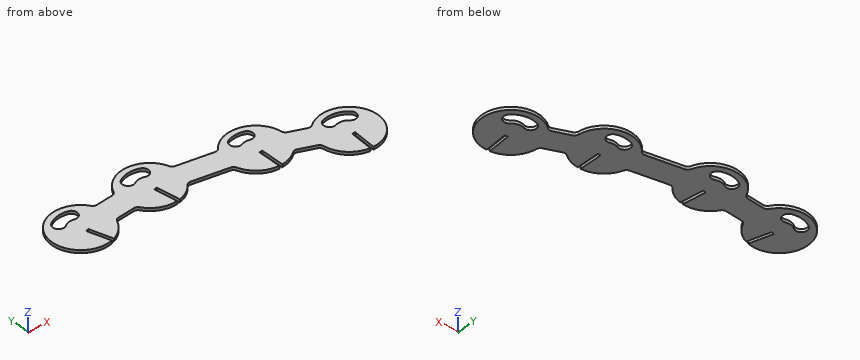
from build123d import *

# Parameters (mm, degrees)
BOSS_EXTRUDE1_DEPTH = 0.8128


with BuildPart() as part:
    # Sketch4 → Boss-Extrude1 (new body)
    with BuildSketch(Plane.XY):
        with BuildLine():
            ThreePointArc((93.949424924, 80.553749396), (79.926578404, 79.107244128), (89.201071756, 68.490447291))
            Line((89.201071756, 68.490447291), (87.379404166, 74.562672592))
            Line((87.379404166, 74.562672592), (87.768664768, 74.679450772))
            Line((87.768664768, 74.679450772), (88.157925371, 74.796228953))
            Line((88.157925371, 74.796228953), (89.979592961, 68.724003652))
            ThreePointArc((89.979592961, 68.724003652), (92.683522719, 70.35568471), (94.537210983, 72.912530234))
            ThreePointArc((94.537210983, 72.912530234), (94.965343033, 73.427292247), (95.595760228, 73.652794227))
            Line((95.595760228, 73.652794227), (100.153762821, 74.003409811))
            ThreePointArc((100.153762821, 74.003409811), (100.811251698, 73.876977473), (101.313075076, 73.433750604))
            ThreePointArc((101.313075076, 73.433750604), (104.499077144, 70.639420699), (108.66874425, 69.88260829))
            Line((108.66874425, 69.88260829), (107.772190929, 76.15848154))
            Line((107.772190929, 76.15848154), (108.174506403, 76.215955179))
            Line((108.174506403, 76.215955179), (108.576821877, 76.273428818))
            Line((108.576821877, 76.273428818), (109.473375199, 69.997555568))
            ThreePointArc((109.473375199, 69.997555568), (112.013123253, 70.968780496), (114.076058013, 72.740191859))
            ThreePointArc((114.076058013, 72.740191859), (114.622955908, 73.126429859), (115.290273938, 73.180870175))
            Line((115.290273938, 73.180870175), (124.839494012, 71.390391411))
            ThreePointArc((124.839494012, 71.390391411), (125.441762928, 71.097903494), (125.811592802, 70.539779051))
            ThreePointArc((125.811592802, 70.539779051), (128.535078066, 66.714656664), (132.9436, 65.097910667))
            Line((132.9436, 65.097910667), (132.9436, 71.447910667))
            Line((132.9436, 71.447910667), (133.35, 71.447910667))
            Line((133.35, 71.447910667), (133.7564, 71.447910667))
            Line((133.7564, 71.447910667), (133.7564, 65.097910667))
            ThreePointArc((133.7564, 65.097910667), (136.15889652, 65.601119169), (138.292771811, 66.814290453))
            ThreePointArc((138.292771811, 66.814290453), (138.908022168, 67.078379412), (139.572075423, 66.99288524))
            Line((139.572075423, 66.99288524), (143.735615445, 65.258076898))
            ThreePointArc((143.735615445, 65.258076898), (144.263910207, 64.846759758), (144.509615464, 64.223938699))
            ThreePointArc((144.509615464, 64.223938699), (146.734319899, 59.528365603), (151.386817059, 57.214929481))
            Line((151.386817059, 57.214929481), (151.873839827, 63.546225464))
            Line((151.873839827, 63.546225464), (152.27904277, 63.515056007))
            Line((152.27904277, 63.515056007), (152.684245713, 63.48388655))
            Line((152.684245713, 63.48388655), (152.197222945, 57.152590567))
            ThreePointArc((152.197222945, 57.152590567), (159.92620767, 67.609424733), (147.457228033, 71.298209423))
            ThreePointArc((147.457228033, 71.298209423), (146.84197711, 71.034120487), (146.177923414, 71.119615244))
            Line((146.177923414, 71.119615244), (142.014384371, 72.854423179))
            ThreePointArc((142.014384371, 72.854423179), (141.486089803, 73.265740229), (141.240384561, 73.888561071))
            ThreePointArc((141.240384561, 73.888561071), (135.620274674, 80.630902915), (127.223942036, 78.0723082))
            ThreePointArc((127.223942036, 78.0723082), (126.677044199, 77.68607018), (126.009726211, 77.631629797))
            Line((126.009726211, 77.631629797), (116.460505988, 79.422108589))
            ThreePointArc((116.460505988, 79.422108589), (115.858237072, 79.714596506), (115.488407198, 80.272720949))
            ThreePointArc((115.488407198, 80.272720949), (108.380699585, 85.713306212), (100.725289029, 81.074969792))
            ThreePointArc((100.725289029, 81.074969792), (100.297156978, 80.560207761), (99.666739772, 80.334705773))
            Line((99.666739772, 80.334705773), (95.108737382, 79.984090204))
            ThreePointArc((95.108737382, 79.984090204), (94.451248393, 80.110522482), (93.949424924, 80.553749396))
        make_face()
        with BuildLine():
            ThreePointArc((156.824589095, 69.642224068), (156.857122838, 67.397395778), (154.612294548, 67.364862034))
            ThreePointArc((154.612294548, 67.364862034), (153.086943568, 68.187295725), (151.356947016, 68.08627733))
            ThreePointArc((151.356947016, 68.08627733), (149.336031859, 69.064139502), (150.313894032, 71.085054659))
            ThreePointArc((150.313894032, 71.085054659), (153.773887136, 71.287091449), (156.824589095, 69.642224068))
        make_face(mode=Mode.SUBTRACT)
        with BuildLine():
            ThreePointArc((88.224829537, 79.241098456), (86.773324607, 79.32888397), (85.434920368, 78.760335862))
            ThreePointArc((85.434920368, 78.760335862), (83.215962621, 79.101713977), (83.557340736, 81.320671724))
            ThreePointArc((83.557340736, 81.320671724), (86.234149214, 82.457767939), (89.137159073, 82.282196911))
            ThreePointArc((89.137159073, 82.282196911), (90.201543533, 80.305482915), (88.224829537, 79.241098456))
        make_face(mode=Mode.SUBTRACT)
        with BuildLine():
            ThreePointArc((106.29439622, 80.496669822), (104.112009419, 81.023452843), (104.63879244, 83.205839644))
            ThreePointArc((104.63879244, 83.205839644), (107.474111012, 84.119642581), (110.41416195, 83.639884632))
            ThreePointArc((110.41416195, 83.639884632), (111.261217621, 81.560747987), (109.182080975, 80.713692316))
            ThreePointArc((109.182080975, 80.713692316), (107.712055506, 80.953571291), (106.29439622, 80.496669822))
        make_face(mode=Mode.SUBTRACT)
        with BuildLine():
            ThreePointArc((132.117919025, 75.951192316), (130.038782379, 76.798247987), (130.88583805, 78.877384632))
            ThreePointArc((130.88583805, 78.877384632), (133.106309101, 79.370322273), (135.358046314, 79.049138943))
            ThreePointArc((135.358046314, 79.049138943), (136.362069471, 77.041092628), (134.354023157, 76.037069471))
            ThreePointArc((134.354023157, 76.037069471), (133.228154551, 76.197661136), (132.117919025, 75.951192316))
        make_face(mode=Mode.SUBTRACT)
    extrude(amount=BOSS_EXTRUDE1_DEPTH)


solid = part.part
Read the model definition and answer for the solid it produces. Units are mm, in the model's axes. Round coordinates to 2 decimals unless told otherwise and drop trailing zeros. Write each loop counter-clockwise with the first axis right and the second up, starting at its lowest first coordinate (ties: lowest second). Pieces come first, ordered by that corner, then holes. Notation, with made-up numbers: (87, -4.5) - (95, -4.5) arc R21 ccw to (95, 19.5) - close; hole circle Ø11 at (-15, 14.5). An arc over 180 degrees is marked (long way). Use a Markdown table: item, result.
(1) The part is cut by section B-B (z = 0.65). State how many separate pieces and enclosed holes the cut face has, then the cut area to 3 significant figures.
Reported:
| item | result |
|---|---|
| separate pieces | 1 |
| enclosed holes | 4 |
| area | 817 mm2 |
(2) The part is cut by section A-A (x = 92.5). Write down the section's boundary in (y, z), then the cut area to 3 significant figures.
Reported:
| item | result |
|---|---|
| outline | (70.19, 0) - (82.21, 0) - (82.21, 0.81) - (70.19, 0.81) - close |
| area | 9.77 mm2 |
(3) Straight lines are drawn through the part: line 1 along X through (y, z) = (81.75, 0.2); line 2 along X through (y, z) = (62.25, 0.3); line 3 along X through (y, z) = (74.5, 0.4). For each, find the intervals that lie inside material, in ascending order. Write a range as [from, to].
Reported:
| item | result |
|---|---|
| line 1 | [81.64, 84.23], [89.92, 92.99], [101.07, 103.88], [111.33, 114.83] |
| line 2 | [144.99, 151.77], [152.59, 159.81] |
| line 3 | [79.56, 87.4], [88.25, 108.01], [108.83, 141.15] |
